Design review of the part built by this model. Coordinates are the model's own, in mm. Face numbers are marked on the shaded views. A direction names the side the tool comes from. Give positions to 0.01 mm unless a question says otherwise; leave off trailing zeros. Loops run counter-clockwise (first coordinate to the right, second up) from the corner with the lowest first, then second, coordinate; pieces in that order, holes last.
from build123d import *

# Parameters (mm, degrees)
BOSS_EXTRUDE1_DEPTH = 27
SHELL1_START        = 2
SHELL1_DEPTH        = 23


# Read off the part's stored shape, not the designer's step: Shell1
with BuildPart() as part:
    # Sketch1 → Boss-Extrude1 (new body)
    with BuildSketch(Plane.XY):
        with BuildLine():
            Line((45, 0), (-45, 0))
            Line((-45, 0), (-41, -12))
            ThreePointArc((-41, -12), (-21.353939388, -3.317135008), (0, -1))
            ThreePointArc((0, -1), (21.353939388, -3.317135008), (41, -12))
            Line((41, -12), (45, 0))
        make_face()
    extrude(amount=BOSS_EXTRUDE1_DEPTH)

    # Shell1 outline → Shell1 (cut)
    with BuildSketch(Plane.XY.offset(SHELL1_START)):
        with BuildLine():
            Line((-42.891814893, 0), (-39.90071559, -8.97329791))
            ThreePointArc((-39.90071559, -8.97329791), (-28.159071544, -3.3851069), (-15.603788395, 0))
            Line((-15.603788395, 0), (-42.891814893, 0))
        make_face()
        with BuildLine():
            Line((42.891814893, 0), (15.603788395, 0))
            ThreePointArc((15.603788395, 0), (28.159071544, -3.3851069), (39.90071559, -8.97329791))
            Line((39.90071559, -8.97329791), (42.891814893, 0))
        make_face()
    extrude(amount=SHELL1_DEPTH, mode=Mode.SUBTRACT)


solid = part.part
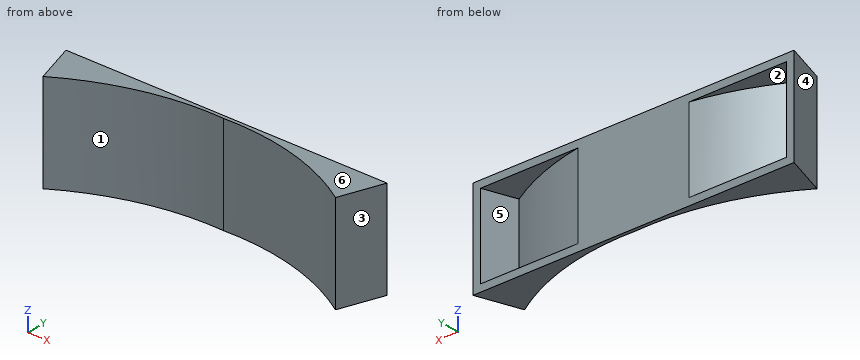
Q1. Take a section at A-A (y = -6.5). Give the boundary of the cut face in (x, z), plus the area to 3 significant figures.
Results:
outline: (-42.83, 0) - (-30.59, 0) - (-30.59, 27) - (-42.83, 27) - close; (30.59, 0) - (42.83, 0) - (42.83, 27) - (30.59, 27) - close; hole (-40.73, 2) - (-35.36, 2) - (-35.36, 25) - (-40.73, 25) - close; hole (35.36, 2) - (40.73, 2) - (40.73, 25) - (35.36, 25) - close
area: 414 mm2
Q2. Draft analysis for pull direction X (two halves, no side actions). For the marked faces 4, 5 and 6, state which applies: pulls with the +X half, pulls with the -X half, needs draft (parallel to the pull), parting line crosses it, or undercut.
Results:
face 4: pulls with the -X half
face 5: undercut
face 6: needs draft
Q3. Take a section at C-C (x = -32). Give the boundary of the cut face in (y, z).
Results:
outline: (-7.12, 0) - (0, 0) - (0, 2) - (-4.93, 2) - (-4.93, 25) - (0, 25) - (0, 27) - (-7.12, 27) - close
Q4. Take a section at D-D (y = -2.75). Give the boundary of the cut face in (x, z), plus the area to 3 significant figures.
Results:
outline: (-44.08, 0) - (-19.09, 0) - (-19.09, 27) - (-44.08, 27) - close; (19.09, 0) - (44.08, 0) - (44.08, 27) - (19.09, 27) - close; hole (-41.98, 2) - (-26.37, 2) - (-26.37, 25) - (-41.98, 25) - close; hole (26.37, 2) - (41.98, 2) - (41.98, 25) - (26.37, 25) - close
area: 632 mm2
Q5. Take a section at B-B (z = 10.5). Give the boundary of the cut face in (x, y), plus the area to 3 significant figures.
Results:
outline: (-45, 0) - (-41, -12) arc R70 cw to (0, -1) arc R70 cw to (41, -12) - (45, 0) - (42.89, 0) - (39.9, -8.97) arc R72 ccw to (15.6, 0) - (-15.6, 0) arc R72 ccw to (-39.9, -8.97) - (-42.89, 0) - close
area: 189 mm2
Q6. Insertion check: pin 1 (6 mm diameter, centred on x = 5.5, z = 16.5, fed in from -Y); pin 2 (5 mm diameter, centred on y = -9, z = 21, fed in from +X); pin 3 (6 mm diameter, centred on y = -8, z = 5.5, fed in from -X); pin 4 (2.5 mm diameter, centred on x = -25.5, y = -6.5, fed in from +Z). Each pin has a flat end and moves straight along its axis. Give the tip position at first contact, or say it passes through.
Results:
pin 1: stops at y = -1.13
pin 2: stops at x = 42.83
pin 3: stops at x = -43.33
pin 4: passes through
Q7. Wall thickness on line 1 (Z direction, x = -35, y = -4.5); line 2 (X direction, y = -7.25, z = 13.75); line 3 (Y direction, x = -4.5, z = 5.75): over which ranges is each line inside the solid? List them lowest first.
Results:
line 1: z = 0 to 2, 25 to 27
line 2: x = -42.58 to -40.48, -36.82 to -32.29, 32.29 to 36.82, 40.48 to 42.58
line 3: y = -0.94 to 0
Q8. Tool access review of the marked faces 1, 2 and 3: name each direction out of +Z, -Z, +X, -X, +Y, -Y from which nothing blocks a thin tool from reaching the whole face with its end or side.
Results:
face 1: +Z, -Z, -Y
face 2: +Y
face 3: +Z, -Z, +X, -Y
